Check sheet for the modelled part. Datum: model origin and axes. Units: mm. Round coordinates to 2 decimals unless told otherwise and drop trailing zeros. Order: outer loops, then holes, each group sorted by start corner. A loop starts at its lowest first (then second) coordinate and runs counter-clockwise, first axis right, second up. Notation, with made-up numbers: (64.25, 64.5) -> (108.25, 64.5) arc R24 ccw to (108.25, 74.5) -> close; hole circle Ø11 at (66, 6.25). An arc over 180 degrees is marked (long way). Answer in a Markdown table with one row per item.
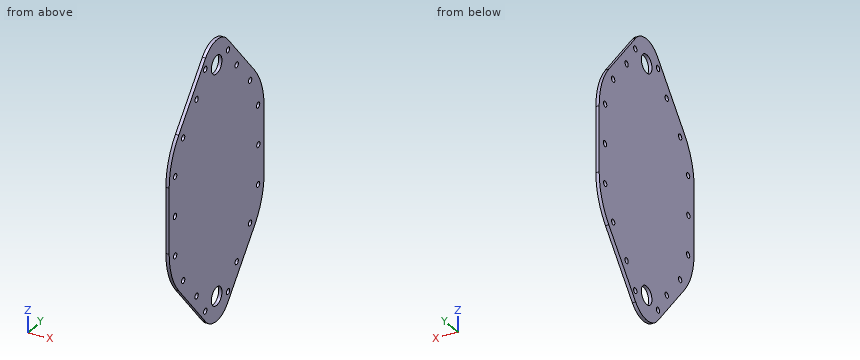
from build123d import *

# Parameters (mm, degrees)
SKETCH1_R               = 19.05
BOSS_EXTRUDE1_DEPTH     = 2.54
CUT_EXTRUDE3_DEPTH      = 125.81903469
CUT_EXTRUDE3_DEPTH_BACK = 125.81903469
SKETCH4_R               = 2.159
SKETCH5_R               = 6.985
CUT_EXTRUDE4_DEPTH      = 6.35


with BuildPart() as part:
    # Sketch1 → Boss-Extrude1 (new body)
    with BuildSketch(Plane(origin=(0, 0, 0), x_dir=(0, 0, -1), z_dir=(1, 0, 0))):
        with BuildLine():
            Line((25.4, 62.611), (-25.4, 62.611))
            ThreePointArc((-25.4, 62.611), (-43.71389723, 59.350669702), (-59.777434529, 49.970298982))
            Line((-59.777434529, 49.970298982), (-101.281034529, 14.478))
            ThreePointArc((-101.281034529, 14.478), (-80.929937509, 17.302618411), (-69.85, 0))
            ThreePointArc((-69.85, 0), (-80.929937509, -17.302618411), (-101.281034529, -14.478))
            Line((-101.281034529, -14.478), (-59.777434529, -49.970298982))
            ThreePointArc((-59.777434529, -49.970298982), (-43.71389723, -59.350669702), (-25.4, -62.611))
            Line((-25.4, -62.611), (25.4, -62.611))
            ThreePointArc((25.4, -62.611), (43.699078076, -59.34404997), (59.737214243, -49.946847768))
            Line((59.737214243, -49.946847768), (101.269374674, -14.487973703))
            ThreePointArc((101.269374674, -14.487973703), (69.85, -7.706e-06), (101.269379322, 14.48794821))
            Line((101.269379322, 14.48794821), (59.737230268, 49.9468356))
            ThreePointArc((59.737230268, 49.9468356), (43.699087699, 59.344046737), (25.4, 62.611))
        make_face()
        with Locations((88.9, -1.0762e-05)):
            Circle(SKETCH1_R)
        with Locations((-88.9, 0)):
            Circle(SKETCH1_R)
    extrude(amount=BOSS_EXTRUDE1_DEPTH)

    # Sketch4 → Cut-Extrude3 (cut, two sides: drawn at the far end of the back side and taken through both)
    with BuildSketch(Plane(origin=(2.54, 0, 0), x_dir=(0, 0, -1), z_dir=(1, 0, 0)).offset(-CUT_EXTRUDE3_DEPTH_BACK)):
        with Locations((-30.48, 54.706186836)):
            Circle(SKETCH4_R)
        with Locations((-54.833341451, 44.171983407)):
            Circle(SKETCH4_R)
        with Locations((54.789478539, 44.151652011)):
            Circle(SKETCH4_R)
        with Locations((30.478659799, 54.70517335)):
            Circle(SKETCH4_R)
        with Locations((-75.580981084, 26.429391704)):
            Circle(SKETCH4_R)
        with Locations((75.555553066, 26.422208316)):
            Circle(SKETCH4_R)
        with Locations((0, 54.991)):
            Circle(SKETCH4_R)
        with Locations((-92.852981084, 14.999391704)):
            Circle(SKETCH4_R)
        with Locations((92.827553066, 14.992208316)):
            Circle(SKETCH4_R)
        with Locations((92.827553066, -14.992208316)):
            Circle(SKETCH4_R)
        with Locations((75.555553066, -26.422208316)):
            Circle(SKETCH4_R)
        with Locations((54.789478539, -44.151652011)):
            Circle(SKETCH4_R)
        with Locations((30.478659799, -54.70517335)):
            Circle(SKETCH4_R)
        with Locations((0, -54.991)):
            Circle(SKETCH4_R)
        with Locations((-30.48, -54.706186836)):
            Circle(SKETCH4_R)
        with Locations((-54.833341451, -44.171983407)):
            Circle(SKETCH4_R)
        with Locations((-75.580981084, -26.429391704)):
            Circle(SKETCH4_R)
        with Locations((-92.852981084, -14.999391704)):
            Circle(SKETCH4_R)
    extrude(amount=CUT_EXTRUDE3_DEPTH + CUT_EXTRUDE3_DEPTH_BACK, mode=Mode.SUBTRACT)

    # Sketch5 → Cut-Extrude4 (cut)
    with BuildSketch(Plane(origin=(2.54, 0, 0), x_dir=(0, 0, -1), z_dir=(1, 0, 0))):
        with Locations((-88.9, 0)):
            Circle(SKETCH5_R)
        with Locations((88.9, -1.0762e-05)):
            Circle(SKETCH5_R)
    extrude(amount=-CUT_EXTRUDE4_DEPTH, mode=Mode.SUBTRACT)


solid = part.part
Item 1: Cross-section at B-B (z = 30.48). Record the boundary of the cut face in (x, y).
Result sheet:
| item | result |
|---|---|
| outline | (0, -62.37) -> (2.54, -62.37) -> (2.54, -56.87) -> (0, -56.87) -> close; (0, -52.55) -> (2.54, -52.55) -> (2.54, 52.55) -> (0, 52.55) -> close; (0, 56.87) -> (2.54, 56.87) -> (2.54, 62.37) -> (0, 62.37) -> close |
Item 2: Depth check by flat-ended pin: P1, Ø1, axis at x = 2, z = -82, coming from the +Y side. Enter the tip coordinate at first touch or a pass-through.
Result sheet:
| item | result |
|---|---|
| P1 | stops at y = 31.37 |
Item 3: Cross-section at A-A (x = 0.9). State how many separate pieces and enclosed holes the cut face has, and give its area (3 significant figures).
Result sheet:
| item | result |
|---|---|
| separate pieces | 1 |
| enclosed holes | 20 |
| area | 19,500 mm^2 |
Item 4: Scan lines: line 1 (Z direction, x = 2.2, y = -25.5); line 2 (Z direction, x = 1.75, y = -3.5); line 3 (Z direction, x = 1.15, y = -54.5). Record each from-to range of solid material in increasing order. Write a range as [from, to].
Result sheet:
| item | result |
|---|---|
| line 1 | z = [-88.37, -77.51], [-73.6, 73.63], [77.53, 88.39] |
| line 2 | z = [-107.63, -94.94], [-82.86, 82.86], [94.94, 107.63] |
| line 3 | z = [-53.54, -32.63], [-28.33, -2.1], [2.1, 28.33], [32.63, 53.6] |
